Geometry: see drawing. Coordinates: mm, zero at the bounding-box minimum. Give positions to 0.01 mm unless a question says otherwise; leave off trailing zeros. Write each loop counter-clockwise with the first axis right and the second up, starting at its lowest first coordinate (ties: lowest second). Pieces come first, ordered by that corner, then holes. Notation, with made-up numbers: (83.25, 50) -> (108.25, 50) arc R13 cw to (108.25, 71) -> close; hole circle Ø10 at (39, 23.25). An arc over 180 degrees is marked (long way). Use one line per item in the form item = value. Start each with the question number.
(1) Cut plane A-A, the plane z = 71.5. Output: boundary loops of the cut face in (x, y), and give its area (3 significant figures).
(2) Cut plane B-B, the plane y = 22.5. Output: boundary loops of the cut face in (x, z), and give its area (3 significant figures).
(3) Material intervals for line 1 along Z through (x, y) = (549.5, 10.5); line 2 along X through (y, z) = (3, 34.5); line 3 along X through (y, z) = (6, 36.5), sorted ascending. Write a range as from..to.
(4) First-contact query: P1, Ø1.5, axis at y = 11.5, z = 74.5, coming from the -X side; P2, Ø11.5, axis at y = 18.5, z = 74, coming from the -X side; P3, Ø6, axis at y = 33, z = 14.5, coming from the +X side. Flat tips, straight axial feed; report the tip coordinate or a pass-through.
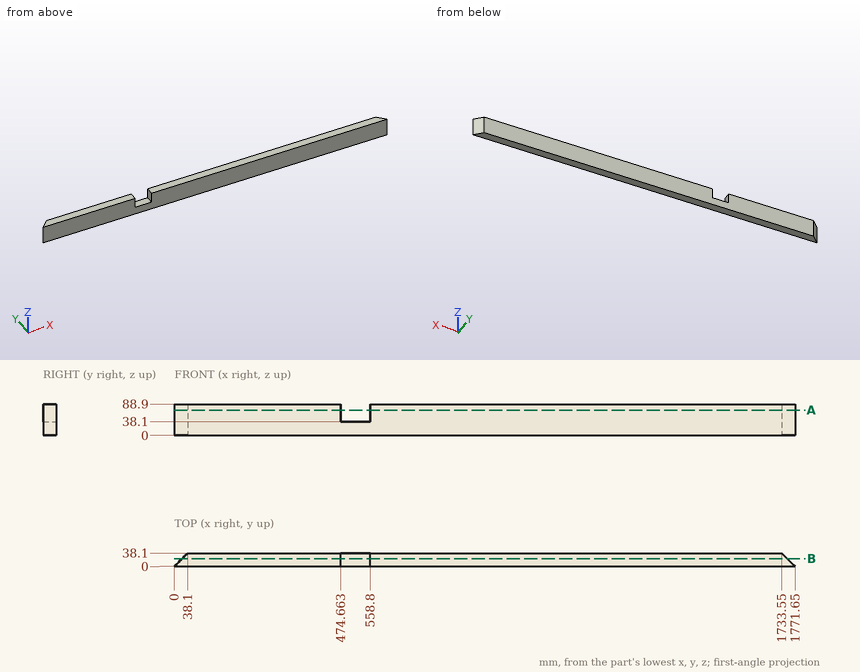
Geometry says:
q1.outline = (0, 0) -> (474.66, 0) -> (474.66, 38.1) -> (38.1, 38.1) -> close; (558.8, 0) -> (1771.65, 0) -> (1733.55, 38.1) -> (558.8, 38.1) -> close
q1.area = 62,800 mm^2
q2.outline = (22.5, 0) -> (1749.15, 0) -> (1749.15, 88.9) -> (558.8, 88.9) -> (558.8, 38.1) -> (474.66, 38.1) -> (474.66, 88.9) -> (22.5, 88.9) -> close
q2.area = 149,000 mm^2
q3.line_1 = 0..38.1
q3.line_2 = 3..1768.65
q3.line_3 = 6..1765.65
q4.P1 = 10.75
q4.P2 = 12.75
q4.P3 = 1741.65
